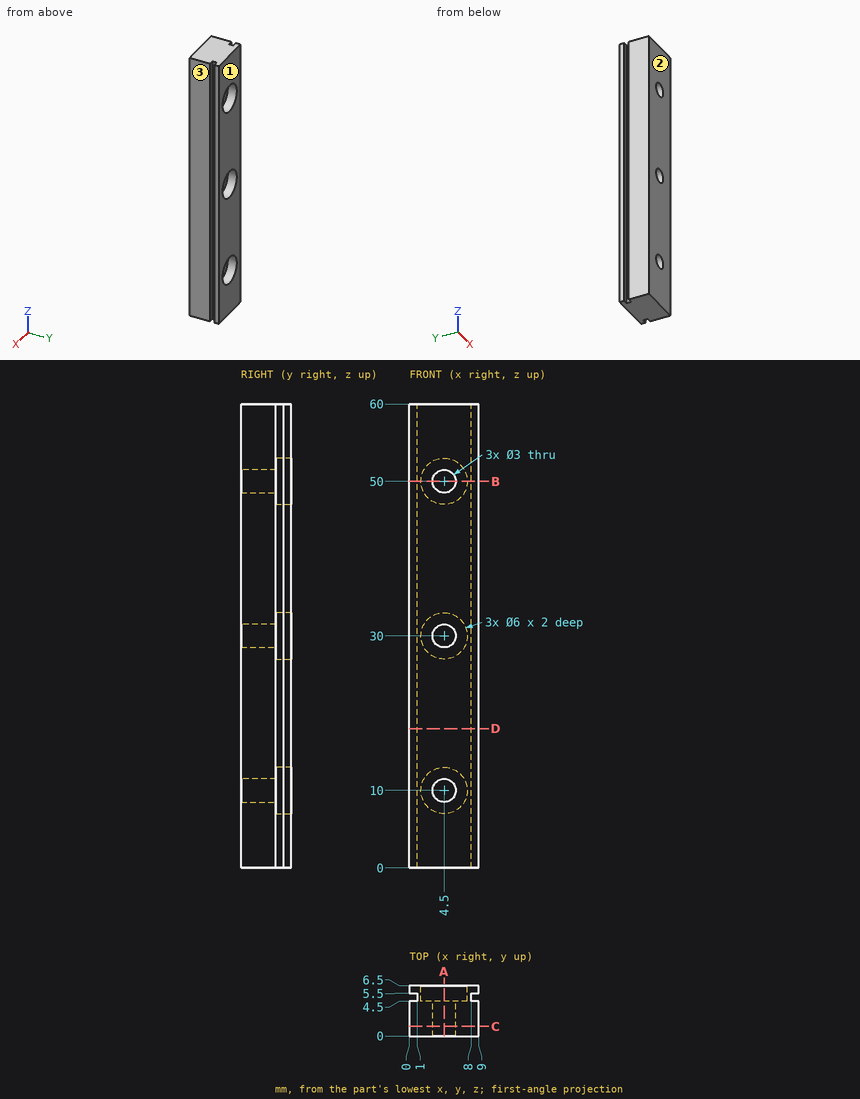
The figure shows three views and two pictorial views of one solid part (mm, origin at its lowest corner). Answer the questions. Give positions to 0.01 mm unless a question says otherwise; leave off trailing zeros. Loops run counter-clockwise (first coordinate to the right, second up) from the corner with the lowest first, then second, coordinate; pieces in that order, holes last. Notation, with made-up numbers: M 6,82 L 22,82 A20 cw 22,111 Z; hole C 83.25,9.25 d1. An arc over 180 degrees is marked long. Write each question's results on one line, items separated by ' | '.
1. Section B-B on z = 50 is taken. Give the vertices of the cut face in (x, y).
Values:
outline: M 0,0 L 3,0 L 3,4.5 L 1.5,4.5 L 1.5,6.5 L 0,6.5 L 0,5.5 L 1,5.5 L 1,4.5 L 0,4.5 Z; M 6,0 L 9,0 L 9,4.5 L 8,4.5 L 8,5.5 L 9,5.5 L 9,6.5 L 7.5,6.5 L 7.5,4.5 L 6,4.5 Z
2. Section C-C on y = 1.25 is taken. Give the vertices of the cut face in (x, z).
Values:
outline: M 0,0 L 9,0 L 9,60 L 0,60 Z; hole C 4.5,10 d3; hole C 4.5,30 d3; hole C 4.5,50 d3
3. Section D-D on z = 18 is taken. Give the vertices of the cut face in (x, y), plus the area to 3 significant figures.
Values:
outline: M 0,0 L 9,0 L 9,4.5 L 8,4.5 L 8,5.5 L 9,5.5 L 9,6.5 L 0,6.5 L 0,5.5 L 1,5.5 L 1,4.5 L 0,4.5 Z | area: 56.5 mm^2
4. Section A-A on x = 4.5 is taken. Give the vertices of the cut face in (y, z).
Values:
outline: M 0,0 L 6.5,0 L 6.5,7 L 4.5,7 L 4.5,8.5 L 0,8.5 Z; M 0,11.5 L 4.5,11.5 L 4.5,13 L 6.5,13 L 6.5,27 L 4.5,27 L 4.5,28.5 L 0,28.5 Z; M 0,31.5 L 4.5,31.5 L 4.5,33 L 6.5,33 L 6.5,47 L 4.5,47 L 4.5,48.5 L 0,48.5 Z; M 0,51.5 L 4.5,51.5 L 4.5,53 L 6.5,53 L 6.5,60 L 0,60 Z
5. The mould has two halves that part along Y. Classify the marked faces 1, 2 and 3: pulls with the +Y half, pulls with the -Y half, needs draft (parallel to the pull), parting line crosses it, or undercut.
Values:
face 1: pulls with the +Y half | face 2: pulls with the -Y half | face 3: needs draft
6. Straight lines are drawn through the part: line 1 (X direction, y = 2.2, z = 50); line 2 (Y direction, x = 0.5, z = 34); line 3 (X direction, y = 5.2, z = 50). For each, find the intervals that lie inside material, in ascending order. Write a range as [from, to].
Values:
line 1: x = [0, 3], [6, 9] | line 2: y = [0, 4.5], [5.5, 6.5] | line 3: x = [1, 1.5], [7.5, 8]
7. Given pin 1 (2.5 mm diameter, centred on x = 4.5, z = 10, fed in from +Y); pin 2 (1.8 mm diameter, centred on x = 4.5, z = 29, fed in from +Y), each flat-ended and moving along its own axis, determine where each tip first touches the part or whether it passes through.
Values:
pin 1: passes through | pin 2: stops at y = 4.5
